Check sheet for the modelled part. Datum: model origin and axes. Units: mm. A direction names the side the tool comes from. Round coordinates to 2 decimals unless told otherwise and drop trailing zeros. Write each loop counter-clockwise with the first axis right and the second up, starting at its lowest first coordinate (ties: lowest second). Pieces come first, ordered by that corner, then holes.
Item 1: Material ranges on line 1 (Z direction, x = 2.3, y = 0) (3 decimals); line 2 (Y direction, x = 1.1, z = 0), recorded low to high.
Item 2: Tool access check on faces 1 (the flat face through (0.255, 1, 2)), 2 (the flat face through (2.245, -1, 2)). Record the directions out of +Z, -Z, +X, -X, +Y, -Y that give a thin tool (end or side, any length) a straight path to the whole face; none if there is none.
Item 3: Cross-section at C-C on x = 0.85. Enter the section's corners in (y, z), plus the area to 3 significant figures.
Item 4: Release check for a two-part mould opening along Z. For faces 3 (the cylindrical face through (1, -3, 0)), 4 (the cylindrical face through (1.23, -1.5, -0.07)) record: +Z half, -Z half, draft (parallel to the pull), parting line (faces both ways), or undercut.
Item 5: Go/stop test with flat-tipped pins: pin 1 Ø1.5 at (x, y) = (0.5, 2.5) entering from -Z; pin 2 Ø1 at (x, z) = (1, 2) entering from -Y; pin 3 Ø1 at (x, y) = (0.5, -1) entering from -Z. Record where each tip stops, or that it passes through.
from build123d import *


with BuildPart() as part:
    # 草图1 → 旋转1 (revolve)
    with BuildSketch(Plane(origin=(0, 0, 0), x_dir=(-1, 0, 0), z_dir=(0, 0, -1))):
        with BuildLine():
            Line((0, 2.075), (-0.255, 2.075))
            Line((-0.255, 2.075), (-0.255, 2.7))
            Line((-0.255, 2.7), (0, 2.7))
            Line((0, 2.7), (0, 2.92))
            ThreePointArc((0, 2.92), (-0.023431458, 2.976568542), (-0.08, 3))
            Line((-0.08, 3), (-2.42, 3))
            ThreePointArc((-2.42, 3), (-2.476568542, 2.976568542), (-2.5, 2.92))
            Line((-2.5, 2.92), (-2.5, 2.7))
            Line((-2.5, 2.7), (-2.245, 2.7))
            Line((-2.245, 2.7), (-2.245, 2.075))
            Line((-2.245, 2.075), (-2.5, 2.075))
            Line((-2.5, 2.075), (-2.5, 1.58))
            ThreePointArc((-2.5, 1.58), (-2.476568542, 1.523431458), (-2.42, 1.5))
            Line((-2.42, 1.5), (-0.08, 1.5))
            ThreePointArc((-0.08, 1.5), (-0.023431458, 1.523431458), (0, 1.58))
            Line((0, 1.58), (0, 2.075))
        make_face()
    revolve(axis=Axis((2.5, 0, 0), (-1, 0, 0)))


solid = part.part
Response values:
1. line 1: z = -3 to -2.7, -2.075 to -1.5, 1.5 to 2.075, 2.7 to 3
1. line 2: y = -3 to -1.5, 1.5 to 3
2. face 1: -X
2. face 2: +X
3. outline: circle Ø6 at (0, 0); hole circle Ø3 at (0, 0)
3. area: 21.2 mm2
4. face 3: parting line
4. face 4: undercut
5. pin 1: stops at z = -2.44
5. pin 2: stops at y = -2.6
5. pin 3: stops at z = -2.96
